Design review of the part shown in the three views and the two pictorial views. Dimensions are in mm from the part's minimum x, y and z. A direction names the side the tool comes from. Coordinates: 2 decimals unless noted, no trailing zeros. Loops run counter-clockwise (first coordinate to the right, second up) from the corner with the lowest first, then second, coordinate; pieces in that order, holes last.
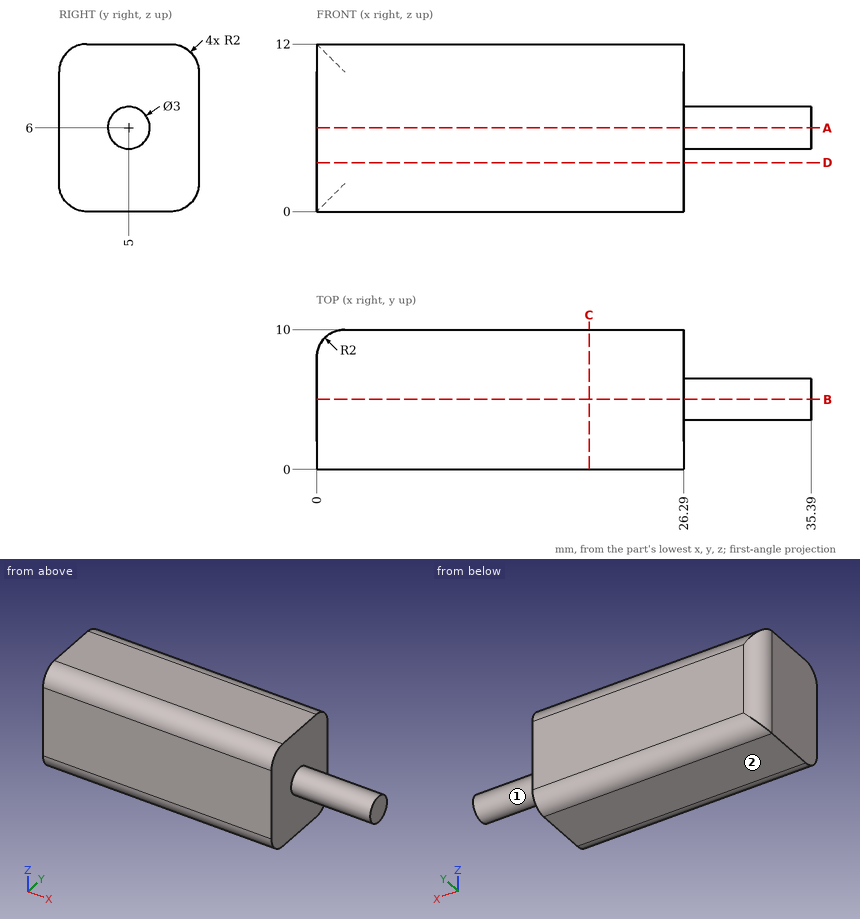
Q1. Consider section A-A (z = 6). State the section outline as (x, y) points.
Q2. Wall thickness on probe 1 along X at (y, z) = (6.25, 1.5); probe 2 along Z at (x, y) = (12.5, 8.5); probe 3 along Y at (x, z) = (22.5, 11): over which ranges is each line inside the solid? List them lowest first.
Q3. Consider section B-B (y = 5). State the section outline as (x, z) points.
Q4. Consider section D-D (z = 3.5). State the section outline as (x, y) points.
Q5. Consider section C-C (x = 19.5). State the section outline as (y, z) points, then the cut area to 3 significant figures.
Q6. Machinability: for the marked faces 1 and 2, which of the approach directions +Z, -Z, +X, -X, +Y, -Y give a long, thin tool a straight path to every point of the face, cutting with its end or side? Answer none if there is none.
Model answer:
1. outline: (0, 0) - (26.29, 0) - (26.29, 3.5) - (35.39, 3.5) - (35.39, 6.5) - (26.29, 6.5) - (26.29, 10) - (2, 10) arc R2 ccw to (0, 8) - close
2. probe 1: x = 0 to 26.29
2. probe 2: z = 0.06 to 11.94
2. probe 3: y = 0.27 to 9.73
3. outline: (0, 0) - (26.29, 0) - (26.29, 4.5) - (35.39, 4.5) - (35.39, 7.5) - (26.29, 7.5) - (26.29, 12) - (0, 12) - close
4. outline: (0, 0) - (26.29, 0) - (26.29, 10) - (2, 10) arc R2 ccw to (0, 8) - close
5. outline: (0, 2) arc R2 ccw to (2, 0) - (8, 0) arc R2 ccw to (10, 2) - (10, 10) arc R2 ccw to (8, 12) - (2, 12) arc R2 ccw to (0, 10) - close
5. area: 117 mm2
6. face 1: +X
6. face 2: -Z, +X, -X, +Y, -Y
